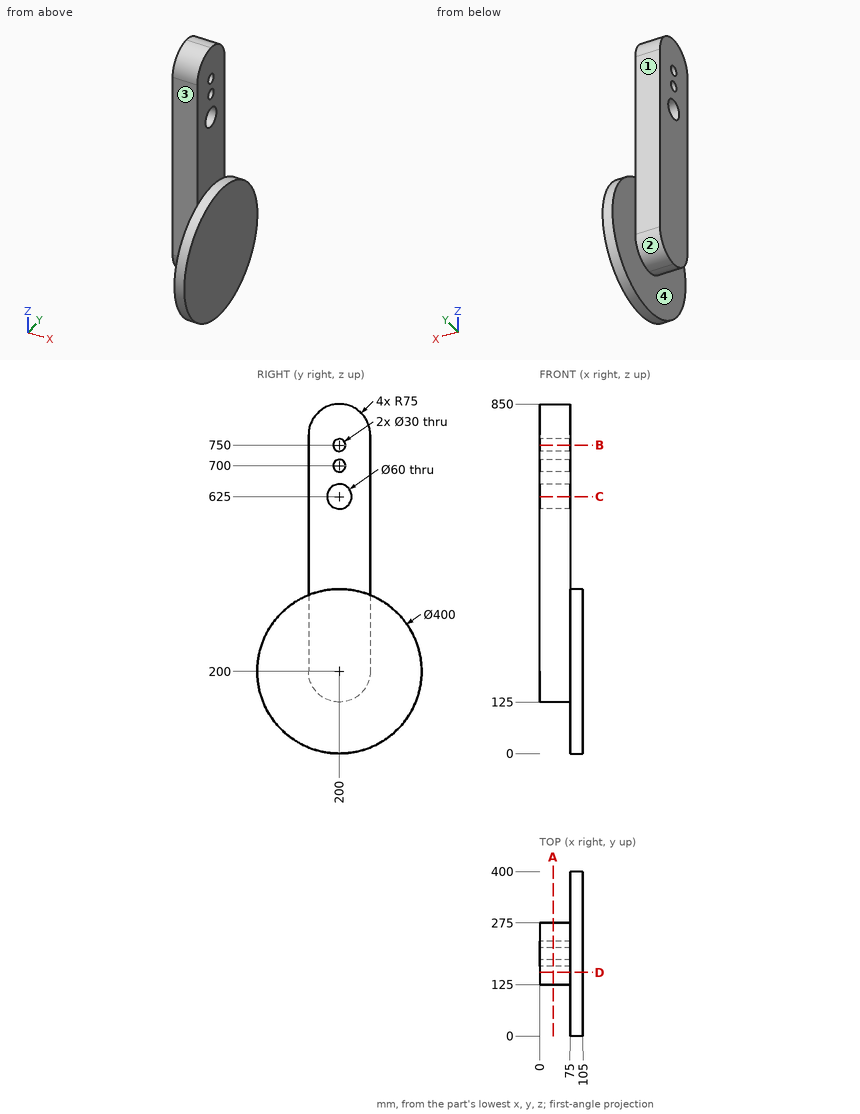
Source: three-view drawing plus pictorial views. Frame: mm from the lowest corner of the part. A direction names the side the tool comes from. Give positions to 0.01 mm unless a question says otherwise; leave off trailing zeros. Write each loop counter-clockwise with the first axis right and the second up, starting at its lowest first coordinate (ties: lowest second). Pieces come first, ordered by that corner, then holes. Notation, with made-up numbers: (88, 6) - (129, 6) arc R26 ccw to (129, 36) - close; hole circle Ø8 at (14.5, 51). An arc over 180 degrees is marked (long way). Write item = value, one per line. Start each with the question number.
1. Section query A-A, the plane x = 32.5. Count the separate pieces of the cut face and the enclosed holes in it, then the cut area to 3 significant figures.
2. First-contact query: pin 1 Ø1.5 at (x, y) = (42.5, 189.5) entering from -Z; pin 2 Ø2 at (x, z) = (59, 706.5) entering from +Y; pin 3 Ø2 at (x, z) = (47, 434) entering from -Y. Flat tips, straight axial feed; report the tip coordinate or a pass-through.
3. Section query D-D, the plane y = 155. Output: boundary loops of the cut face in (x, z).
4. Section query B-B, the plane z = 750. Output: boundary loops of the cut face in (x, y).
5. Ray query, L1, parallel to Z at x = 55, y = 200; L2, parallel to Y at x = 17.5, z = 750; L3, parallel to Y at x = 48, z = 277.5. Return the intervals inside material, ascending.
6. Section query C-C, the plane z = 625. Output: boundary loops of the cut face in (x, y).
7. Access query for the marked faces 1, 2, 3 and 4. Directions: +Z, -Z, +X, -X, +Y, -Y. A direction counts if a zero-diameter tool reaches every point of the face in a straight line with its end or side. Return the directions, or none.
Check sheet entries:
q1.separate_pieces = 1
q1.enclosed_holes = 3
q1.area = 99,700 mm2
q2.pin_1 = 125.64
q2.pin_2 = 275
q2.pin_3 = 125
q3.outline = (0, 140) - (75, 140) - (75, 5.13) - (105, 5.13) - (105, 394.87) - (75, 394.87) - (75, 835) - (0, 835) - close
q4.outline = (0, 125) - (75, 125) - (75, 185) - (0, 185) - close; (0, 215) - (75, 215) - (75, 275) - (0, 275) - close
q5.L1 = 125 to 595, 655 to 685, 715 to 735, 765 to 850
q5.L2 = 125 to 185, 215 to 275
q5.L3 = 125 to 275
q6.outline = (0, 125) - (75, 125) - (75, 170) - (0, 170) - close; (0, 230) - (75, 230) - (75, 275) - (0, 275) - close
q7.face_1 = +Z, -Z, -X, +Y
q7.face_2 = -Z, -X, +Y
q7.face_3 = +Z, -Z, -X, -Y
q7.face_4 = -Z, -X
